Read the model definition and answer for the solid it produces. Units are mm, in the model's axes. A direction names the side the tool comes from. Coordinates: 2 decimals unless noted, no trailing zeros. Write each loop counter-clockwise with the first axis right and the second up, starting at its lowest first coordinate (ties: lowest second). Pieces come first, ordered by that corner, then holes.
(1) Section B-B on z = 9.75 is taken. Write down the section's boundary in (x, y).
(2) Which of the six approach directions +Z, -Z, +X, -X, +Y, -Y give full straight-line access (tool end or side, diameter ignored) to faces 1 (the flat face through (1, 34, 0)), 2 (the flat face through (8, 21, 16.8))?
(3) Given pin 1 (1 mm diameter, centred on y = 30, z = 14, fed in from -X); pin 2 (12 mm diameter, centred on x = 11, y = -22, fed in from +Z), each flat-ended and moving along its own axis, determine where each tip first touches the part or whether it passes through.
(4) The mould has two halves that part along Y. Classify faces 3 (the flat face through (7.457, 21.031, 16.455)), 4 (the flat face through (1, 34, 20)), 5 (the flat face through (9.825, 19.16, 9.86)), 6 (the flat face through (5, 79.3, 10)): +Y half, -Y half, draft (parallel to the pull), parting line (faces both ways), or undercut.
(5) Section A-A on x = -10 is taken. Write down the section's boundary in (y, z), then the cut area to 3 significant figures.
(6) Section C-C on y = 72 is taken. Write down the section's boundary in (x, z).
(7) Find the intervals of material crossed by probe 1 along Z at (x, y) = (1, 66); probe 2 along Y at (x, z) = (-6, 3.5); probe 3 along X at (y, z) = (58.5, 2.75), in increasing order.
(8) Section D-D on x = 7 is taken. Write down the section's boundary in (y, z), then the cut area to 3 significant figures.
from build123d import *

# Parameters (mm, degrees)
F1_DEPTH = 20
F2_T     = -0.7
F3_W     = 121.1464474762
F3_H     = 0.7
F4_DEPTH = 2


with BuildPart() as f1:
    # F0 (on Top) → F1 (new body)
    with BuildSketch(Plane.XY):
        Polygon((22.5, 80), (-12.5, 80), (-12.5, -40), (-2.5, -40), align=None)
    extrude(amount=F1_DEPTH)

    # F2
    f2_openings = [f1.faces().sort_by_distance(p)[0] for p in [
        (-12.5, 20, 10),
    ]]
    offset(amount=F2_T, openings=f2_openings)

    # F3 (on face) → F4 (join)
    with BuildSketch(Plane(origin=(4.9053959025, -1.0219574797, 0), x_dir=(-0.2039542541, -0.9789804197, 0), z_dir=(-0.9789804197, 0.2039542541, 0))):
        with Locations((-21.4733176025, 16.45)):
            Rectangle(F3_W, F3_H)
    extrude(amount=F4_DEPTH)


solid = f1.part
Response:
1. outline: (-12.5, -40) - (-2.5, -40) - (22.5, 80) - (-12.5, 80) - (-12.5, 79.3) - (21.64, 79.3) - (-3.07, -39.3) - (-12.5, -39.3) - close
2. face 1: -Z, +X, -X, +Y, -Y
2. face 2: -X
3. pin 1: stops at x = 11.26
3. pin 2: passes through
4. face 3: undercut
4. face 4: draft
4. face 5: -Y half
4. face 6: undercut
5. outline: (-40, 0) - (80, 0) - (80, 20) - (-40, 20) - close; hole (-39.3, 0.7) - (79.3, 0.7) - (79.3, 19.3) - (-39.3, 19.3) - close
5. area: 194 mm2
6. outline: (-12.5, 0) - (20.83, 0) - (20.83, 20) - (-12.5, 20) - (-12.5, 19.3) - (20.12, 19.3) - (20.12, 16.8) - (18.08, 16.8) - (18.08, 16.1) - (20.12, 16.1) - (20.12, 0.7) - (-12.5, 0.7) - close
7. probe 1: z = 0 to 0.7, 19.3 to 20
7. probe 2: y = -40 to -39.3, 79.3 to 80
7. probe 3: x = 17.31 to 18.02
8. outline: (5.6, 0) - (80, 0) - (80, 20) - (5.6, 20) - close; hole (9.03, 0.7) - (79.3, 0.7) - (79.3, 19.3) - (9.03, 19.3) - (9.03, 16.8) - (18.84, 16.8) - (18.84, 16.1) - (9.03, 16.1) - close
8. area: 188 mm2
